Autodesk Inventor part; units mm, degrees
ref_plane "YZ Plane" through (0, 0, 0) normal (1, 0, 0) x (0, 1, 0)
ref_plane "XZ Plane" through (0, 0, 0) normal (0, 1, 0) x (-1, 0, 0)
ref_plane "XY Plane" through (0, 0, 0) normal (0, 0, 1) x (1, 0, 0)
sketch "Sketch1" plane through (0, 0, 0) normal (1, 0, 0) x (0, 1, 0)
  line L0 (0, 0) -> (-25.4, 0)
  line L1 (-25.4, 0) -> (-25.4, 25.4)
  line L2 (-25.4, 25.4) -> (0, 25.4)
  line L3 (0, 25.4) -> (0, 0)
  line L4 (-3.175, 3.175) -> (-22.225, 3.175)
  line L5 (-22.225, 3.175) -> (-22.225, 22.225)
  line L6 (-22.225, 22.225) -> (-3.175, 22.225)
  line L7 (-3.175, 22.225) -> (-3.175, 3.175)
  dimension "d0" = 25.4
  dimension "d1" = 25.4
  dimension "d2" = 19.05
  dimension "d3" = 19.05
  dimension "d4" = 3.175
  dimension "d5" = 3.175
extrude "Extrusion1" add sketch "Sketch1" along normal blind 603.25
sketch "Sketch2" plane through (0, -25.4, 25.4) normal (0, 0, 1) x (1, 0, 0)
  line L0 (0, 0) -> (0, 25.4)
  line L1 (0, 0) -> (603.25, 0)
  line L2 (603.25, 25.4) -> (603.25, 0)
  line L3 (0, 25.4) -> (603.25, 25.4)
  point P0 (12.7, 12.7)
  point P1 (301.625, 12.7)
  point P2 (590.55, 12.7)
  dimension "d8" = 12.7
  dimension "d9" = 12.7
  dimension "d10" = 12.7
  dimension "d11" = 12.7
  dimension "d12" = 12.7
  dimension "d13" = 301.625
hole "Hole1" at (12.7, -12.7, 25.4) at (301.625, -12.7, 25.4) at (590.55, -12.7, 25.4) direction (0, 0, -1) diameter 6.35 end through all
sketch "Sketch3" plane through (0, -25.4, 0) normal (0, 0, -1) x (-1, 0, 0)
  circle A0 centre (-301.625, 12.7) radius 3.175
  circle A1 centre (-12.7, 12.7) radius 3.175
  circle A2 centre (-590.55, 12.7) radius 3.175
  line L0 (0, 25.4) -> (0, 0)
  line L1 (0, 25.4) -> (-603.25, 25.4)
  line L2 (-603.25, 0) -> (-603.25, 25.4)
  line L3 (0, 0) -> (-603.25, 0)
  circle A3 centre (-12.7, 12.7) radius 3.175
  circle A4 centre (-12.7, 12.7) radius 7.9375
  circle A5 centre (-301.625, 12.7) radius 7.9375
  circle A6 centre (-590.55, 12.7) radius 3.175
  circle A7 centre (-590.55, 12.7) radius 7.9375
  dimension "d21" = 15.875
  dimension "d22" = 15.875
  dimension "d23" = 15.875
extrude "Extrusion2" cut sketch "Sketch3" against normal blind 12.7 contours A4 | A5 | A7
sketch "Sketch4" plane through (0, -25.4, 25.4) normal (0, 0, 1) x (1, 0, 0)
  circle A0 centre (301.625, 12.7) radius 3.175
  circle A1 centre (12.7, 12.7) radius 3.175
  circle A2 centre (590.55, 12.7) radius 3.175
  line L0 (0, 0) -> (0, 25.4)
  line L1 (0, 0) -> (603.25, 0)
  line L2 (603.25, 25.4) -> (603.25, 0)
  line L3 (0, 25.4) -> (603.25, 25.4)
  point P0 (38.1, 12.7)
  point P1 (565.15, 12.7)
  dimension "d26" = 12.7
  dimension "d27" = 38.1
  dimension "d28" = 12.7
  dimension "d29" = 38.1
hole "Hole2" at (38.1, -12.7, 25.4) at (565.15, -12.7, 25.4) direction (0, 0, -1) diameter 6.35 end through all
properties part number "1x1 support horizontal"
Part model, mm, in its own coordinate system. A direction names the side the tool comes from. Round coordinates to 2 decimals unless told otherwise and drop trailing zeros. Loops run counter-clockwise (first coordinate to the right, second up) from the corner with the lowest first, then second, coordinate; pieces in that order, holes last.
1. Flat gauge pin, fed straight in: pin 1 (1.5 mm diameter, centred on y = -11, z = 21, fed in from -X). Where does the tip first touch, or does it go through?
Solutions:
pin 1: passes through
2. Slice it at A-A (z = 9.5). Give the cut face in (x, y) (3 decimals).
Solutions:
outline: (0, -25.4) - (603.25, -25.4) - (603.25, -22.225) - (0, -22.225) - close; (0, -3.175) - (603.25, -3.175) - (603.25, 0) - (0, 0) - close
3. Slice it at B-B (x = 89). Give the cut face in (y, z) (3 decimals).
Solutions:
outline: (-25.4, 0) - (0, 0) - (0, 25.4) - (-25.4, 25.4) - close; hole (-22.225, 3.175) - (-3.175, 3.175) - (-3.175, 22.225) - (-22.225, 22.225) - close
4. 3-axis set-ups, long thin cutter, end or side, ignore diameter. For faces 5 (the face through (309.555, -12.351, 1.565)), 6 (the face through (297, -21, 0)), 7 (the face through (297, -21, 3.175)): which of +Z, -Z, +X, -X, +Y, -Y reach the whole face in a straight line?
Solutions:
face 5: -Z
face 6: -Z, +X, -X, +Y, -Y
face 7: +X, -X
5. Drill centre lines: line 1 along X through (y, z) = (-12.7, 23.85) (3 decimals); line 2 along Y through (x, z) = (565.15, 23.4) (3 decimals); line 3 along Y through (x, z) = (102, 15.5) (3 decimals). Where is each one in solid material? Low to high.
Solutions:
line 1: x = 0 to 9.525, 15.875 to 34.925, 41.275 to 298.45, 304.8 to 561.975, 568.325 to 587.375, 593.725 to 603.25
line 2: y = -25.4 to -15.875, -9.525 to 0
line 3: y = -25.4 to -22.225, -3.175 to 0
6. Two-plate mould, pull along Z, no slides. Class faces 1 (the face through (297, 0, 13)), 2 (the face through (297, -13, 22.225)), 3 (the face through (297, -13, 25.4)), 4 (the face through (297, -3.175, 13)): pulls with the +Z half, pulls with the -Z half, needs draft (parallel to the pull), parting line crosses it, or undercut.
Solutions:
face 1: needs draft
face 2: undercut
face 3: pulls with the +Z half
face 4: undercut
